from build123d import *

# Parameters (mm, degrees)
SKETCH1_W            = 155
SKETCH1_H            = 55
BOSS_EXTRUDE1_DEPTH  = 5
SKETCH2_W            = 30
SKETCH2_H            = 25
CUT_EXTRUDE2_DEPTH   = 5
SKETCH3_W            = 5
SKETCH3_H            = 55
BOSS_EXTRUDE2_DEPTH  = 40
SKETCH10_W           = 55
SKETCH10_H           = 5
SKETCH14_W           = 125
SKETCH14_H           = 30
BOSS_EXTRUDE7_DEPTH  = 5
BOSS_EXTRUDE8_REACH  = 107
SKETCH16_W           = 30
SKETCH16_H           = 5
SKETCH19_W           = 4
SKETCH19_H           = 55
BOSS_EXTRUDE9_DEPTH  = 40
CUT_EXTRUDE4_DEPTH   = 125
SKETCH18_R           = 1.75
CUT_EXTRUDE5_DEPTH   = 5
SKETCH20_W           = 38
SKETCH20_H           = 16
CUT_EXTRUDE6_DEPTH   = 5
FILLET1_R            = 5
SKETCH21_W           = 5
SKETCH21_H           = 20
BOSS_EXTRUDE10_DEPTH = 36
CUT_EXTRUDE7_DEPTH   = 4
SKETCH23_W           = 36
SKETCH23_H           = 10.5
CUT_EXTRUDE8_DEPTH   = 5
FILLET2_R            = 2
SKETCH24_W           = 20
SKETCH24_H           = 23
CUT_EXTRUDE9_DEPTH   = 5
FILLET3_R            = 2
CHAMFER1_SIZE        = 45
CHAMFER1_SIZE2       = 20.983844617
FILLET4_R            = 10
FILLET5_R            = 10


with BuildPart() as part:
    # Sketch1 → Boss-Extrude1 (new body)
    with BuildSketch(Plane(origin=(0, 0, 0), x_dir=(1, 0, 0), z_dir=(0, 1, 0))):
        Rectangle(SKETCH1_W, SKETCH1_H)
    extrude(amount=BOSS_EXTRUDE1_DEPTH)

    # Sketch2 → Cut-Extrude2 (cut)
    with BuildSketch(Plane(origin=(0, 5, 0), x_dir=(1, 0, 0), z_dir=(0, 1, 0))):
        with Locations((-62.5, 15)):
            Rectangle(SKETCH2_W, SKETCH2_H)
    extrude(amount=-CUT_EXTRUDE2_DEPTH, mode=Mode.SUBTRACT)

    # Sketch3 → Boss-Extrude2 (add)
    with BuildSketch(Plane.XZ):
        with Locations((-45, 0)):
            Rectangle(SKETCH3_W, SKETCH3_H)
    extrude(amount=BOSS_EXTRUDE2_DEPTH)

    # Sweep1: sweep along a path in Sketch9
    with BuildLine(Plane.XY.offset(27.5)) as sweep1_path:
        Line((187.5, -70), (142.672413793, -22.931034483))
        ThreePointArc((142.672413793, -22.931034483), (112.952736872, -2.276947298), (77.5, 5))
    # Sketch10 → Sweep1 (sweep)
    with BuildSketch(Plane(origin=(77.5, 0, 0), x_dir=(0, 0, -1), z_dir=(1, 0, 0))):
        with Locations((0, 2.5)):
            Rectangle(SKETCH10_W, SKETCH10_H)
    sweep(path=sweep1_path.line)

    # Sketch14 → Boss-Extrude7 (add)
    with BuildSketch(Plane(origin=(0, -40, 0), x_dir=(1, 0, 0), z_dir=(0, 1, 0))):
        with Locations((20, 12.5)):
            Rectangle(SKETCH14_W, SKETCH14_H)
    extrude(amount=BOSS_EXTRUDE7_DEPTH)

    # Boss-Extrude8: up to this face of the body (flat: up to its plane)
    boss_extrude8_end = Plane(part.part.faces().sort_by_distance((161.465517241, -49.913793103, 0))[0])
    # Sketch16 → Boss-Extrude8 (add, up to the picked face)
    with BuildSketch(Plane(origin=(82.5, 0, 0), x_dir=(0, 0, -1), z_dir=(1, 0, 0)), mode=Mode.PRIVATE) as boss_extrude8_sk1:
        with Locations((12.5, -37.5)):
            Rectangle(SKETCH16_W, SKETCH16_H)
    boss_extrude8_tool1 = split(extrude(boss_extrude8_sk1.sketch, amount=BOSS_EXTRUDE8_REACH, mode=Mode.PRIVATE), bisect_by=boss_extrude8_end, keep=Keep.BOTH, mode=Mode.PRIVATE)
    add(boss_extrude8_tool1.solids().sort_by_distance((82.5, -37.5, -12.5))[0])

    # Sketch19 → Boss-Extrude9 (add)
    with BuildSketch(Plane.XZ):
        with Locations((75.5, 0)):
            Rectangle(SKETCH19_W, SKETCH19_H)
        with Locations((35.5, 0)):
            Rectangle(SKETCH19_W, SKETCH19_H)
        with Locations((-4.5, 0)):
            Rectangle(SKETCH19_W, SKETCH19_H)
    extrude(amount=BOSS_EXTRUDE9_DEPTH)

    # Sketch17 → Cut-Extrude4 (cut)
    with BuildSketch(Plane.ZY.offset(47.5)):
        Polygon((27.5, 0), (2.5, -40), (27.5, -40), align=None)
    extrude(amount=-CUT_EXTRUDE4_DEPTH, mode=Mode.SUBTRACT)

    # Sketch18 → Cut-Extrude5 (cut)
    with BuildSketch(Plane(origin=(0, -35, 0), x_dir=(1, 0, 0), z_dir=(0, 1, 0))):
        with Locations((-30.5, 17)):
            Circle(SKETCH18_R)
        with Locations((69.5, 17)):
            Circle(SKETCH18_R)
    extrude(amount=-CUT_EXTRUDE5_DEPTH, mode=Mode.SUBTRACT)

    # Sketch20 → Cut-Extrude6 (cut)
    with BuildSketch(Plane(origin=(0, -35, 0), x_dir=(1, 0, 0), z_dir=(0, 1, 0))):
        with Locations((100.5, 9.5)):
            Rectangle(SKETCH20_W, SKETCH20_H)
    extrude(amount=-CUT_EXTRUDE6_DEPTH, mode=Mode.SUBTRACT)

    # Fillet1
    fillet1_edges = [part.edges().sort_by_distance(p)[0] for p in [
        (81.5, -37.5, -1.5),
        (81.5, -37.5, -17.5),
        (119.5, -37.5, -17.5),
        (119.5, -37.5, -1.5),
    ]]
    fillet(fillet1_edges, radius=FILLET1_R)

    # Sketch21 → Boss-Extrude10 (add)
    with BuildSketch(Plane.ZY.offset(-73.5)):
        with Locations((7.5, -10)):
            Rectangle(SKETCH21_W, SKETCH21_H)
    extrude(amount=BOSS_EXTRUDE10_DEPTH)

    # Sketch22 → Cut-Extrude7 (cut)
    with BuildSketch(Plane.ZY.offset(-73.5)):
        Polygon((10, -28), (27.5, 0), (10, 0), align=None)
    extrude(amount=-CUT_EXTRUDE7_DEPTH, mode=Mode.SUBTRACT)

    # Sketch23 → Cut-Extrude8 (cut)
    with BuildSketch(Plane.XZ):
        with Locations((55.5, 15.25)):
            Rectangle(SKETCH23_W, SKETCH23_H)
    extrude(amount=-CUT_EXTRUDE8_DEPTH, mode=Mode.SUBTRACT)

    # Fillet2
    fillet2_edges = [part.edges().sort_by_distance(p)[0] for p in [
        (37.5, -7.5, 10),
        (73.5, 2.5, 10),
        (73.5, 2.5, 20.5),
        (37.5, 2.5, 20.5),
    ]]
    fillet(fillet2_edges, radius=FILLET2_R)

    # Sketch24 → Cut-Extrude9 (cut)
    with BuildSketch(Plane.XZ):
        with Locations((15.5, -16)):
            Rectangle(SKETCH24_W, SKETCH24_H)
    extrude(amount=-CUT_EXTRUDE9_DEPTH, mode=Mode.SUBTRACT)

    # Fillet3
    fillet3_edges = [part.edges().sort_by_distance(p)[0] for p in [
        (-77.5, 2.5, -2.5),
        (-47.5, -17.5, -27.5),
        (-47.5, 2.5, -2.5),
        (5.5, 2.5, -4.5),
        (5.5, 2.5, -27.5),
        (25.5, 2.5, -27.5),
        (25.5, 2.5, -4.5),
    ]]
    fillet(fillet3_edges, radius=FILLET3_R)

    # Chamfer1
    chamfer1_edges = [part.edges().sort_by_distance(p)[0] for p in [
        (185.689655172, -71.724137931, 27.5),
    ]]
    chamfer1_side = [part.faces().sort_by_distance(p)[0] for p in [
        (111.864070979, -4.817167716, 27.5),
    ]]
    chamfer(chamfer1_edges, length=CHAMFER1_SIZE, length2=CHAMFER1_SIZE2, reference=chamfer1_side[0])

    # Fillet4
    fillet4_edges = [part.edges().sort_by_distance(p)[0] for p in [
        (185.689655172, -71.724137931, 6.516155383),
        (154.655172414, -39.137931034, 27.5),
    ]]
    fillet(fillet4_edges, radius=FILLET4_R)

    # Fillet5
    fillet5_edges = [part.edges().sort_by_distance(p)[0] for p in [
        (185.689655172, -71.724137931, -27.5),
    ]]
    fillet(fillet5_edges, radius=FILLET5_R)


solid = part.part
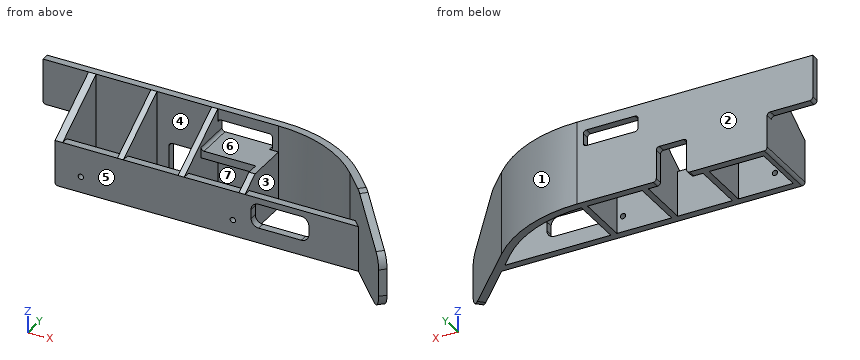
For this review, take the finished solid that the model builds, in its own axes (mm). Face numbers are marked on the shaded views. A direction names the side the tool comes from. Give positions to 0.01 mm unless a question says otherwise; leave off trailing zeros. Order: outer loops, then holes, each group sorted by start corner. A loop starts at its lowest first (then second) coordinate and runs counter-clockwise, first axis right, second up. Notation, with made-up numbers: (70, -11) - (108, -11) arc R29 ccw to (108, 9) - close; hole circle Ø2 at (2.25, -13). An arc over 180 degrees is marked (long way). Answer as a JSON object with one key per item and string values. Group by question number.
Item 1: Take a section at C-C on x = 111. Give the boundary of the cut face in (y, z), and give its area (3 significant figures).
Item 2: Machinability: for the marked faces 4, 5, 6 and 7, which of the approach directions +Z, -Z, +X, -X, +Y, -Y give a long, thin tool a straight path to every point of the face, cutting with its end or side? Answer none if there is none.
Item 3: Draft analysis for pull direction X (two halves, no side actions). For the marked faces 1, 2 and 3, state which applies: pulls with the +X half, pulls with the -X half, needs draft (parallel to the pull), parting line crosses it, or undercut.
Item 4: Clearance check with flat-ended pins moving along their axes: pin 1 Ø3 at (y, z) = (-24, 11) entering from -X; pin 2 Ø8 at (x, z) = (137, -19.5) entering from -Y; pin 3 Ø9 at (x, z) = (95.5, -12) entering from -Y. State where each tip first meets the part, or that it passes through.
Item 5: Take a section at A-A on x = -37. Give the boundary of the cut face in (y, z).
Item 6: Take a section at B-B on y = -15.5. Give the boundary of the cut face in (x, z), and give its area (3 significant figures).
Item 7: Wall thickness on line 1 along Z through (x, y) = (69.5, -37.6); line 2 along X through (y, z) = (-38.9, -17); line 3 along X through (y, z) = (-36, -17): over which ranges is each line inside the solid? List them lowest first.
Reported:
{
 "1": {"outline": "(-40, -27.5) - (-35, -27.5) - (-35, -17.5) - (-40, -17.5) - close; (-40, -1.5) - (-35, -1.5) - (-35, 2.5) - (-40, 2.5) - close; (-6.88, -27.5) - (-1.47, -27.5) - (-1.47, 27.5) - (-6.88, 27.5) - close", "area": "368 mm^2"},
 "2": {"face 4": "+Z, -Z", "face 5": "+Z, -Z, -X, -Y", "face 6": "-Y", "face 7": "-Z"},
 "3": {"face 1": "pulls with the +X half", "face 2": "needs draft", "face 3": "undercut"},
 "4": {"pin 1": "x = -47.5", "pin 2": "y = -40", "pin 3": "y = -3.03"},
 "5": {"outline": "(-40, -27.5) - (-35, -27.5) - (-35, 2.5) - (-40, 2.5) - close; (0, -27.5) - (5, -27.5) - (5, 27.5) - (0, 27.5) - close"},
 "6": {"outline": "(-47.5, -25.5) arc R2 ccw to (-45.5, -27.5) - (-42.5, -27.5) - (-42.5, 17.81) - (-47.5, 17.81) - close; (-6.5, -27.5) - (-2.5, -27.5) - (-2.5, 17.81) - (-6.5, 17.81) - close; (33.5, -27.5) - (37.5, -27.5) - (37.5, 5) - (73.5, 5) - (73.5, -27.5) - (77.5, -27.5) - (77.5, 10) - (39.5, 10) arc R2 cw to (37.5, 12) - (37.5, 17.81) - (33.5, 17.81) - close; (126.44, -27.5) - (134.68, -27.5) - (134.68, 27.5) - (126.44, 27.5) - close", "area": "1,370 mm^2"},
 "7": {"line 1": "-27.5 to -18.75, -15.25 to 2.5", "line 2": "-47.5 to -32.25, -28.75 to 67.75, 71.25 to 84.32, 116.68 to 157.88", "line 3": "-47.5 to -32.25, -28.75 to 67.75, 71.25 to 84.32, 116.68 to 155.12"}
}
